Can you work these out from the model? Positions are in its coordinate system, mm. Face numbers are marked on the shaded views. A direction names the side the tool comes from. Coordinates: 2 decimals unless noted, no trailing zeros. Order: outer loops, then holes, each group sorted by start corner. A loop starts at its lowest first (then second) coordinate and runs counter-clockwise, first axis right, second up. Notation, with made-up numbers: M 37,-31.5 L 56,-31.5 A17 ccw 56,-24.5 Z; hole C 22,-15 d5. An arc over 180 degrees is marked long. Answer as CSV lines item,"result". Start each with the question number.
1. If we section it at A-A (z = 5): List the corners of the cut face in (x, y) for me.
2. I need wall thicknesses on line 1 along Z through (x, y) = (9.5, 0.8); line 2 along X through (y, z) = (12.5, 17.25). Which ranges of each line are inside material? Lowest first, please. Write a range as from..to.
3. If we section it at B-B (x = 9.5): List the corners of the cut face in (y, z) for me.
4. If we section it at C-C (x = 14.25): List the corners of the cut face in (y, z) for me.
5. If we mould it in two halves opening along X, with no side actions, what happens to the marked faces 3, 4, 5 and 6? For each: released by +X, released by -X, zero draft, split by the parting line, or undercut.
6. On a 3-axis mill with a long thin cutter (end or side, diameter ignored), from which of +Z, -Z, +X, -X, +Y, -Y can I reach the whole of each face in a straight line? I mean the marked faces 1 and 2. Say none if no direction works.
7. Will these pins go through, and if not, where does the flat tip stop? pin 1 (5 mm diameter, centred on x = 4.5, z = 20.5, fed in from -Y); pin 2 (3 mm diameter, centred on x = 15, y = 12, fed in from -Z).
```python
from build123d import *

# Parameters (mm, degrees)
ESBO_O1_W                = 19
ESBO_O1_H                = 19
RESSALTO_EXTRUS_O1_DEPTH = 30
CASCA1_T                 = -1
ESBO_O2_R                = 1.65
CORTE_EXTRUS_O1_DEPTH    = 20


with BuildPart() as part:
    # Esboço1 → Ressalto-extrusão1 (new body)
    with BuildSketch(Plane.XY):
        with Locations((9.5, 9.5)):
            Rectangle(ESBO_O1_W, ESBO_O1_H)
    extrude(amount=RESSALTO_EXTRUS_O1_DEPTH)

    # Casca1
    casca1_openings = [part.faces().sort_by_distance(p)[0] for p in [
        (9.5, 9.5, 30),
        (9.5, 9.5, 0),
    ]]
    offset(amount=CASCA1_T, openings=casca1_openings, kind=Kind.INTERSECTION)

    # Esboço2 → Corte-extrusão1 (cut, through all)
    with BuildSketch(Plane(origin=(0, 19, 0), x_dir=(1, 0, 0), z_dir=(0, 1, 0))):
        with Locations((9.5, -25)):
            Circle(ESBO_O2_R)
        with Locations((9.5, -5)):
            Circle(ESBO_O2_R)
    extrude(amount=-CORTE_EXTRUS_O1_DEPTH, mode=Mode.SUBTRACT)


solid = part.part
```
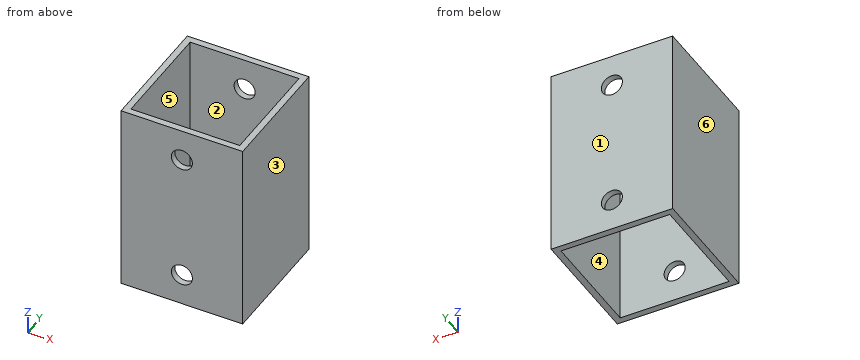
Solved:
1,outline,"M 0,0 L 7.85,0 L 7.85,1 L 1,1 L 1,18 L 7.85,18 L 7.85,19 L 0,19 Z; M 11.15,0 L 19,0 L 19,19 L 11.15,19 L 11.15,18 L 18,18 L 18,1 L 11.15,1 Z"
2,line 1,"0..3.35, 6.65..23.35, 26.65..30"
2,line 2,"0..1, 18..19"
3,outline,"M 0,0 L 1,0 L 1,3.35 L 0,3.35 Z; M 0,6.65 L 1,6.65 L 1,23.35 L 0,23.35 Z; M 0,26.65 L 1,26.65 L 1,30 L 0,30 Z; M 18,0 L 19,0 L 19,3.35 L 18,3.35 Z; M 18,6.65 L 19,6.65 L 19,23.35 L 18,23.35 Z; M 18,26.65 L 19,26.65 L 19,30 L 18,30 Z"
4,outline,"M 0,0 L 1,0 L 1,30 L 0,30 Z; M 18,0 L 19,0 L 19,30 L 18,30 Z"
5,face 3,"released by +X"
5,face 4,"undercut"
5,face 5,"undercut"
5,face 6,"released by -X"
6,face 1,"+Z, -Z, +X, -X, +Y"
6,face 2,"+Z, -Z"
7,pin 1,"y = 0"
7,pin 2,"through"
